```python
from build123d import *

# Parameters (mm, degrees)
EXTRUDE_1_DEPTH          = 1002.5
CUT_EXTRUDE_1_DEPTH      = 1058.062557278
CUT_EXTRUDE_1_DEPTH_BACK = 1058.062557278
SKETCH_2_W               = 400
SKETCH_2_H               = 185
CUT_EXTRUDE_2_DEPTH      = 1058.062557278
CUT_EXTRUDE_2_DEPTH_BACK = 1058.062557278
SKETCH_3_W               = 150
SKETCH_3_H               = 185
CUT_EXTRUDE_3_DEPTH      = 1058.062557278
CUT_EXTRUDE_3_DEPTH_BACK = 1058.062557278
SKETCH_8_W               = 931.455516369
SKETCH_8_H               = 180.779532171
CUT_EXTRUDE_4_DEPTH      = 1058.062557278
CUT_EXTRUDE_4_DEPTH_BACK = 1058.062557278
SKETCH_9_R               = 12


with BuildPart() as part:
    # 草图1 → 凸台-拉伸1 (new body)
    with BuildSketch(Plane(origin=(1027.5, 0, 0), x_dir=(0, 0, -1), z_dir=(1, 0, 0))):
        Polygon((-105, 300), (-105, 180), (-110, 180), (-112.5, 185), (-115, 185), (-115, 165), (-112.5, 165), (-110, 170), (-105, 170), (-105, 50), (-75, 50), (110, 50), (110, 80), (-75, 80), (-75, 260), (-90, 300), align=None)
    extrude(amount=-EXTRUDE_1_DEPTH)

    # 草图2 → 切除-拉伸1 (cut, two sides: drawn at the far end of the back side and taken through both)
    with BuildSketch(Plane(origin=(0, 80, 0), x_dir=(1, 0, 0), z_dir=(0, 1, 0)).offset(-CUT_EXTRUDE_1_DEPTH_BACK)):
        with Locations((526.25, 17.5)):
            Rectangle(SKETCH_2_W, SKETCH_2_H)
    extrude(amount=CUT_EXTRUDE_1_DEPTH + CUT_EXTRUDE_1_DEPTH_BACK, mode=Mode.SUBTRACT)

    # 草图3 → 切除-拉伸2 (cut, two sides: drawn at the far end of the back side and taken through both)
    with BuildSketch(Plane(origin=(0, 80, 0), x_dir=(1, 0, 0), z_dir=(0, 1, 0)).offset(-CUT_EXTRUDE_2_DEPTH_BACK)):
        with Locations((100, 17.5)):
            Rectangle(SKETCH_3_W, SKETCH_3_H)
        with Locations((952.5, 17.5)):
            Rectangle(SKETCH_3_W, SKETCH_3_H)
    extrude(amount=CUT_EXTRUDE_2_DEPTH + CUT_EXTRUDE_2_DEPTH_BACK, mode=Mode.SUBTRACT)

    # 草图8 → 切除-拉伸3 (cut, two sides: drawn at the far end of the back side and taken through both)
    with BuildSketch(Plane(origin=(0, 80, 0), x_dir=(1, 0, 0), z_dir=(0, 1, 0)).offset(-CUT_EXTRUDE_3_DEPTH_BACK)):
        with Locations((511.159415891, 135.389766086)):
            Rectangle(SKETCH_8_W, SKETCH_8_H)
    extrude(amount=CUT_EXTRUDE_3_DEPTH + CUT_EXTRUDE_3_DEPTH_BACK, mode=Mode.SUBTRACT)

    # 草图9 → 切除-拉伸4 (cut, two sides: drawn at the far end of the back side and taken through both)
    with BuildSketch(Plane(origin=(0, 80, 0), x_dir=(1, 0, 0), z_dir=(0, 1, 0)).offset(-CUT_EXTRUDE_4_DEPTH_BACK)):
        with Locations(Location((215, -15, 0), (0, 0, 270))):
            Circle(SKETCH_9_R)
        with Locations(Location((286.25, -15, 0), (0, 0, 270))):
            Circle(SKETCH_9_R)
        with Locations(Location((766.25, -15, 0), (0, 0, 270))):
            Circle(SKETCH_9_R)
        with Locations(Location((837.5, -15, 0), (0, 0, 270))):
            Circle(SKETCH_9_R)
    extrude(amount=CUT_EXTRUDE_4_DEPTH + CUT_EXTRUDE_4_DEPTH_BACK, mode=Mode.SUBTRACT)


solid = part.part
```
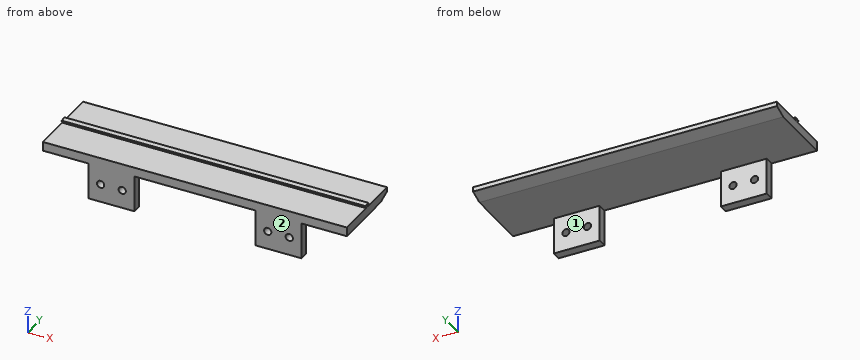
For this review, take the finished solid that the model builds, in its own axes (mm). Face numbers are marked on the shaded views. A direction names the side the tool comes from. Round coordinates to 2 decimals unless told otherwise and drop trailing zeros. Write each loop counter-clockwise with the first axis right and the second up, starting at its lowest first coordinate (ties: lowest second). Pieces come first, ordered by that corner, then holes. Notation, with made-up numbers: (-33, -4) -> (24, -4) arc R22 ccw to (24, 11) -> close; hole circle Ø9 at (88, 23). An arc over 180 degrees is marked (long way). Use one line per item in the form item = value.
Q1. Consider section A-A (z = 15). State the section outline as (x, y) points, then the cut area to 4 significant figures.
Resolved:
outline = (175, 50) -> (203, 50) -> (203, 80) -> (175, 80) -> close; (227, 50) -> (274.25, 50) -> (274.25, 80) -> (227, 80) -> close; (298.25, 50) -> (326.25, 50) -> (326.25, 80) -> (298.25, 80) -> close; (726.25, 50) -> (754.25, 50) -> (754.25, 80) -> (726.25, 80) -> close; (778.25, 50) -> (825.5, 50) -> (825.5, 80) -> (778.25, 80) -> close; (849.5, 50) -> (877.5, 50) -> (877.5, 80) -> (849.5, 80) -> close
area = 6,195 mm²
Q2. Clearance check with flat-ended pins moving along their axes: pin 1 Ø1.5 at (x, y) = (628, 195.5) entering from +Z; pin 2 Ø0.8 at (x, z) = (679.5, 113.5) entering from -Y; pin 3 Ø0.8 at (x, z) = (384.5, 114) entering from +Y. State where each tip first meets the part, or that it passes through.
Resolved:
pin_1 = 105
pin_2 = 165
pin_3 = 185
Q3. To check wall thickness, follow probe 1 along X at (y, z) = (63, 15); probe 2 along Z at (x, y) = (837, 56); probe 3 along X at (y, z) = (70, 41.5). State the ranges of each line that lie inside material, in increasing order. Write a range as from..to.
Resolved:
probe_1 = 175..203, 227..274.25, 298.25..326.25, 726.25..754.25, 778.25..825.5, 849.5..877.5
probe_2 = -45..3.01, 26.99..105
probe_3 = 175..326.25, 726.25..877.5
Q4. Consider section B-B (x = 286.25). State the section outline as (y, z) points.
Resolved:
outline = (50, -45) -> (80, -45) -> (80, 3) -> (50, 3) -> close; (50, 27) -> (80, 27) -> (80, 75) -> (260, 75) -> (300, 90) -> (300, 105) -> (180, 105) -> (180, 110) -> (185, 112.5) -> (185, 115) -> (165, 115) -> (165, 112.5) -> (170, 110) -> (170, 105) -> (50, 105) -> close
Q5. Consider section D-D (x = 444.5). State the section outline as (y, z) points, then the cut area to 3 significant figures.
Resolved:
outline = (50, 75) -> (260, 75) -> (300, 90) -> (300, 105) -> (180, 105) -> (180, 110) -> (185, 112.5) -> (185, 115) -> (165, 115) -> (165, 112.5) -> (170, 110) -> (170, 105) -> (50, 105) -> close
area = 7,340 mm²
Q6. Machinability: for the marked faces 1 and 2, which of the approach directions +Z, -Z, +X, -X, +Y, -Y give a long, thin tool a straight path to every point of the face, cutting with its end or side? Answer none if there is none.
Resolved:
face_1 = -Z, +X, -X, +Y
face_2 = +Z, -Z, +X, -X, -Y
Q7. Consider section C-C (z = -29). State the section outline as (x, y) points.
Resolved:
outline = (175, 50) -> (326.25, 50) -> (326.25, 80) -> (175, 80) -> close; (726.25, 50) -> (877.5, 50) -> (877.5, 80) -> (726.25, 80) -> close
